```python
from build123d import *

# Parameters (mm, degrees)
SKETCH1_R          = 0.5
BASE_FLANGE1_DEPTH = 1


# Sheet-metal steps are written as plain solids
with BuildPart() as part:
    # Sketch1 → Base-Flange1 (new body)
    with BuildSketch(Plane(origin=(0, 0, 0), x_dir=(1, 0, 0), z_dir=(0, 1, 0))):
        with BuildLine():
            Line((-14.178620776, -8), (14.178620776, -8))
            ThreePointArc((14.178620776, -8), (14.789399734, -7.791801152), (15.145851741, -7.253898128))
            Line((15.145851741, -7.253898128), (17.939776994, 3.389626646))
            ThreePointArc((17.939776994, 3.389626646), (17.926022481, 3.944992277), (17.618005902, 4.407318956))
            Line((17.618005902, 4.407318956), (14.829510217, 6.763794182))
            ThreePointArc((14.829510217, 6.763794182), (14.527711383, 6.939093761), (14.184050345, 7))
            Line((14.184050345, 7), (0.25, 7))
            Line((0.25, 7), (0.25, 3))
            Line((0.25, 3), (11.7, 3))
            Line((11.7, 3), (11.7, -3))
            Line((11.7, -3), (-11.7, -3))
            Line((-11.7, -3), (-11.7, 3))
            Line((-11.7, 3), (-0.25, 3))
            Line((-0.25, 3), (-0.25, 7))
            Line((-0.25, 7), (-14.184050345, 7))
            ThreePointArc((-14.184050345, 7), (-14.527711383, 6.939093761), (-14.829510217, 6.763794182))
            Line((-14.829510217, 6.763794182), (-17.618005902, 4.407318956))
            ThreePointArc((-17.618005902, 4.407318956), (-17.926022481, 3.944992277), (-17.939776994, 3.389626646))
            Line((-17.939776994, 3.389626646), (-15.145851741, -7.253898128))
            ThreePointArc((-15.145851741, -7.253898128), (-14.789399734, -7.791801152), (-14.178620776, -8))
        make_face()
        with Locations(Location((-14.2, -7, 0), (0, 0, 270))):
            Circle(SKETCH1_R, mode=Mode.SUBTRACT)
        with Locations(Location((14.2, -7, 0), (0, 0, 270))):
            Circle(SKETCH1_R, mode=Mode.SUBTRACT)
        with Locations(Location((-16.6, 3.643524774, 0), (0, 0, 270))):
            Circle(SKETCH1_R, mode=Mode.SUBTRACT)
        with Locations(Location((16.6, 3.643524774, 0), (0, 0, 270))):
            Circle(SKETCH1_R, mode=Mode.SUBTRACT)
        with Locations(Location((-11.85, 5, 0), (0, 0, 270))):
            Circle(SKETCH1_R, mode=Mode.SUBTRACT)
        with Locations(Location((11.85, 5, 0), (0, 0, 270))):
            Circle(SKETCH1_R, mode=Mode.SUBTRACT)
    extrude(amount=-BASE_FLANGE1_DEPTH)


solid = part.part
```
Check sheet for the modelled part. Datum: model origin and axes. Units: mm. A direction names the side the tool comes from. Give positions to 0.01 mm unless a question says otherwise; leave off trailing zeros. Loops run counter-clockwise (first coordinate to the right, second up) from the corner with the lowest first, then second, coordinate; pieces in that order, holes last. Notation, with made-up numbers: M 57.25,-1 L 115.25,-1 A14 ccw 115.25,3 Z; hole C 7,63.25 d9. An arc over 180 degrees is marked long. Answer in a Markdown table with one row per item.
1) Thickness scan on line 1 (Z direction, x = -1, y = -0.65); line 2 (X direction, y = -0.5, z = -5); line 3 (X direction, y = -0.6, z = 7). Record the ranges inside material, lowest first.
Solutions:
| item | result |
|---|---|
| line 1 | z = -7 to -3, 3 to 8 |
| line 2 | x = -16.92 to -12.35, -11.35 to -0.25, 0.25 to 11.35, 12.35 to 16.92 |
| line 3 | x = -15.21 to -14.7, -13.7 to 13.7, 14.7 to 15.21 |
2) Cross-section at A-A (x = -6). Enter the section's corners in (y, z).
Solutions:
| item | result |
|---|---|
| outline | M -1,-7 L 0,-7 L 0,-3 L -1,-3 Z; M -1,3 L 0,3 L 0,8 L -1,8 Z |
3) Cross-section at C-C (y = -0.5). Enter the section's corners in (x, z).
Solutions:
| item | result |
|---|---|
| outline | M -17.94,-3.39 A1 ccw -17.62,-4.41 L -14.83,-6.76 A1 ccw -14.18,-7 L -0.25,-7 L -0.25,-3 L -11.7,-3 L -11.7,3 L 11.7,3 L 11.7,-3 L 0.25,-3 L 0.25,-7 L 14.18,-7 A1 ccw 14.83,-6.76 L 17.62,-4.41 A1 ccw 17.94,-3.39 L 15.15,7.25 A1 ccw 14.18,8 L -14.18,8 A1 ccw -15.15,7.25 Z; hole C -16.6,-3.64 d1; hole C -14.2,7 d1; hole C -11.85,-5 d1; hole C 11.85,-5 d1; hole C 14.2,7 d1; hole C 16.6,-3.64 d1 |
4) Cross-section at D-D (z = 5). Enter the section's corners in (x, y).
Solutions:
| item | result |
|---|---|
| outline | M -15.74,-1 L 15.74,-1 L 15.74,0 L -15.74,0 Z |
5) Cross-section at B-B (z = -0.75). Enter the section's corners in (x, y), plus the area to 3 significant figures.
Solutions:
| item | result |
|---|---|
| outline | M -17.25,-1 L -11.7,-1 L -11.7,0 L -17.25,0 Z; M 11.7,-1 L 17.25,-1 L 17.25,0 L 11.7,0 Z |
| area | 11.1 mm^2 |
6) Mould release check, pull along Z, two halves, no side actions. Record for faces 1 (the face through (-17.924, -0.493, -3.952)), 2 (the face through (16.523, -0.493, 2.007)), 3 (the face through (0.2, -0.5, 3)): released by +Z, released by -Z, zero draft, split by the parting line, or undercut.
Solutions:
| item | result |
|---|---|
| face 1 | split by the parting line |
| face 2 | released by +Z |
| face 3 | undercut |
7) Tool access check on faces 4 (the face through (-0.25, -0.5, -5)), 5 (the face through (11.7, -0.5, 0)), 6 (the face through (-16.204, -0.493, -5.602)). Record the directions out of +Z, -Z, +X, -X, +Y, -Y that give a thin tool (end or side, any length) a straight path to the whole face; none if there is none.
Solutions:
| item | result |
|---|---|
| face 4 | -Z, +Y, -Y |
| face 5 | +Y, -Y |
| face 6 | -Z, -X, +Y, -Y |
8) Depth check by flat-ended pin: pin 1 (0.5 mm diameter, centred on y = -0.5, z = 0.5, fed in from +X); pin 2 (0.5 mm diameter, centred on y = -0.5, z = -5, fed in from -X); pin 3 (0.5 mm diameter, centred on y = -0.5, z = -5, fed in from +X). Enter the tip coordinate at first touch or a pass-through.
Solutions:
| item | result |
|---|---|
| pin 1 | stops at x = 16.98 |
| pin 2 | stops at x = -17.21 |
| pin 3 | stops at x = 17.21 |
